```python
from build123d import *

# Parameters (mm, degrees)
F0_R     = 40
F1_DEPTH = 85
F2_R     = 20
F3_DEPTH = 88
F4_R     = 5
F5_R     = 33.0630902993
F5_R_2   = 20
F6_DEPTH = 12


with BuildPart() as f1:
    # F0 (on Top) → F1 (new body)
    with BuildSketch(Plane.XY):
        Circle(F0_R)
    extrude(amount=F1_DEPTH)

    # F2 (on face) → F3 (cut)
    with BuildSketch(Plane.XY.offset(85)):
        Circle(F2_R)
    extrude(amount=-F3_DEPTH, mode=Mode.SUBTRACT)

    # F4
    f4_edges = [f1.edges().sort_by_distance(p)[0] for p in [
        (-20, 0, 0),
    ]]
    fillet(f4_edges, radius=F4_R)

    # F5 (on face) → F6 (join)
    with BuildSketch(Plane.XY.offset(85)):
        Circle(F5_R)
        Circle(F5_R_2, mode=Mode.SUBTRACT)
    extrude(amount=F6_DEPTH)


solid = f1.part
```
Input: part model. Units: mm. Frame: model coordinates. A direction names the side the tool comes from. Give positions to 0.01 mm unless a question says otherwise; leave off trailing zeros. Order: outer loops, then holes, each group sorted by start corner. A loop starts at its lowest first (then second) coordinate and runs counter-clockwise, first axis right, second up. Notation, with made-up numbers: M 28.5,68.25 L 56.5,68.25 A27 cw 56.5,84.25 Z; hole C 61,5.5 d8. An arc over 180 degrees is marked long. Return JSON: item names as keys, results as strings.
1) Line query: L1, parallel to Y at x = 0, z = 55; L2, parallel to Y at x = 0, z = 91; L3, parallel to Z at x = -26.5, y = 24. Output: solid intervals per line, ascending. Write a range as [from, to].
Taken from the geometry:
{"L1": "y = [-40, -20], [20, 40]", "L2": "y = [-33.06, -20], [20, 33.06]", "L3": "z = [0, 85]"}
2) Section query A-A on x = 0. Output: boundary loops of the cut face in (y, z), and give its area (3 significant figures).
Taken from the geometry:
{"outline": "M -40,0 L -25,0 A5 ccw -20,5 L -20,97 L -33.06,97 L -33.06,85 L -40,85 Z; M 20,5 A5 ccw 25,0 L 40,0 L 40,85 L 33.06,85 L 33.06,97 L 20,97 Z", "area": "3,700 mm2"}
3) Section query C-C on z = 13. Output: boundary loops of the cut face in (x, y), and give its area (3 significant figures).
Taken from the geometry:
{"outline": "C 0,0 d80; hole C 0,0 d40", "area": "3,770 mm2"}
4) Access query for faces 1 (the face through (-15, 30, 85)), 2 (the face through (-8.67, -39.05, 41.9)). Directions: +Z, -Z, +X, -X, +Y, -Y. A direction counts if a zero-diameter tool reaches every point of the face in a straight line with its end or side. Return the directions, or none.
Taken from the geometry:
{"face 1": "+Z", "face 2": "+Z, -Z"}
5) Section query D-D on x = 28. Output: boundary loops of the cut face in (y, z).
Taken from the geometry:
{"outline": "M -28.57,0 L 28.57,0 L 28.57,85 L 17.58,85 L 17.58,97 L -17.58,97 L -17.58,85 L -28.57,85 Z"}
6) Contact query for flat-ended pins moving along their axis: pin 1 (8 mm diameter, centred on y = -25, z = 20.5, fed in from -X); pin 2 (10 mm diameter, centred on y = 7, z = 84, fed in from +X); pin 3 (10 mm diameter, centred on y = 19.5, z = 52, fed in from -X); pin 4 (24 mm diameter, centred on x = -15.5, y = -2.5, fed in from +Z). Output: stop coordinate, or through.
Taken from the geometry:
{"pin 1": "stops at x = -34.04", "pin 2": "stops at x = 39.95", "pin 3": "stops at x = -37.28", "pin 4": "stops at z = 97"}
